Input: part model. Units: mm. Frame: model coordinates. A direction names the side the tool comes from. Coordinates: 2 decimals unless noted, no trailing zeros. Write each loop counter-clockwise with the first axis right and the second up, starting at its lowest first coordinate (ties: lowest second). Pieces come first, ordered by that corner, then holes. Notation, with made-up numbers: (-18, 84) - (40, 84) arc R27 ccw to (40, 111) - close; hole circle Ø3 at (69.25, 7). An arc over 180 degrees is marked (long way). One line per question, with ' | ' between items. Start each with the question number.
1) Section query A-A on x = 0. Return loops of the section in (y, z).
2) Reachability of faces 1 (the flat face through (15, 65, -67)), 2 (the flat face through (15, 65, 67)), 3 (the flat face through (-15, 65, 67)) from +Z, -Z, +X, -X, +Y, -Y: full face, straight path, thin tool, end or side. Return the list, or none.
3) Section query D-D on x = -34. Return loops of the section in (y, z), and give its area (3 significant figures).
4) Line query: line 1 (Y direction, x = -7, z = -20); line 2 (Y direction, x = -75, z = -63); line 3 (Z direction, x = -0.5, y = 78). Output: solid intervals per line, ascending.
5) Section query B-B on z = 84.5. Return loops of the section in (x, y).
6) Section query C-C on y = -49. Return loops of the section in (x, z).
7) First-contact query: P1, Ø7.5, axis at y = 63, z = 64, coming from the +X side; P2, Ø16.5, axis at y = 70, z = 68.5, coming from the -X side; P3, Ø16.5, axis at y = 61.5, z = -65, coming from the +X side. Flat tips, straight axial feed; report the tip coordinate or a pass-through.
```python
from build123d import *

# Parameters (mm, degrees)
F2_R     = 115
F3_DEPTH = 20


with BuildPart() as f1:
    # F0 (on Right) → F1 (revolve)
    with BuildSketch(Plane.YZ):
        Polygon((-75.25, 100.5), (-75.25, 0), (122.75, 0), (122.75, 10), (75.25, 10), (75.25, 100.5), align=None)
    revolve(axis=Axis((0, 23.75, 0), (0, 1, 0)))

    # F2 (on face) → F3 (cut)
    with BuildSketch(Plane(origin=(0, 75.25, 0), x_dir=(-1, 0, 0), z_dir=(0, 1, 0))):
        Circle(F2_R)
        with BuildLine():
            ThreePointArc((-15, 74.6), (0, 89.6), (15, 74.6))
            Line((15, 74.6), (15, 59.6))
            ThreePointArc((15, 59.6), (43.457796, 43.457796), (59.6, 15))
            Line((59.6, 15), (74.6, 15))
            ThreePointArc((74.6, 15), (89.6, 0), (74.6, -15))
            Line((74.6, -15), (59.6, -15))
            ThreePointArc((59.6, -15), (43.457796, -43.457796), (15, -59.6))
            Line((15, -59.6), (15, -74.6))
            ThreePointArc((15, -74.6), (0, -89.6), (-15, -74.6))
            Line((-15, -74.6), (-15, -59.6))
            ThreePointArc((-15, -59.6), (-43.457796, -43.457796), (-59.6, -15))
            Line((-59.6, -15), (-74.6, -15))
            ThreePointArc((-74.6, -15), (-89.6, 0), (-74.6, 15))
            Line((-74.6, 15), (-59.6, 15))
            ThreePointArc((-59.6, 15), (-43.457796, 43.457796), (-15, 59.6))
            Line((-15, 59.6), (-15, 74.6))
        make_face(mode=Mode.SUBTRACT)
    extrude(amount=-F3_DEPTH, mode=Mode.SUBTRACT)


solid = f1.part
```
Answer key:
1) outline: (-75.25, -100.5) - (55.25, -100.5) - (55.25, -89.6) - (75.25, -89.6) - (75.25, -10) - (122.75, -10) - (122.75, 10) - (75.25, 10) - (75.25, 89.6) - (55.25, 89.6) - (55.25, 100.5) - (-75.25, 100.5) - close
2) face 1: -Z, +X, +Y | face 2: +Z, +X, +Y | face 3: +Z, -X, +Y
3) outline: (-75.25, -94.57) - (55.25, -94.57) - (55.25, -51.2) - (75.25, -51.2) - (75.25, 51.2) - (55.25, 51.2) - (55.25, 94.57) - (-75.25, 94.57) - close | area: 26,700 mm²
4) line 1: -75.25 to 75.25 | line 2: -75.25 to 55.25 | line 3: -9.99 to 9.99
5) outline: (-54.41, -75.25) - (54.41, -75.25) - (54.41, 55.25) - (11.27, 55.25) - (11.27, 75.25) - (-11.27, 75.25) - (-11.27, 55.25) - (-54.41, 55.25) - close
6) outline: circle Ø201 at (0, 0)
7) P1: x = 15 | P2: x = -15 | P3: x = 80.91
